Verification items for the finished model (mm, model axes). A direction names the side the tool comes from. Coordinates: 2 decimals unless noted, no trailing zeros. Loops run counter-clockwise (first coordinate to the right, second up) from the corner with the lowest first, then second, coordinate; pieces in that order, holes last. Notation, with made-up numbers: (-3, 73.25) -> (33, 73.25) arc R26 ccw to (33, 96.25) -> close; hole circle Ø10 at (7.25, 30). An arc over 180 degrees is marked (long way). Write item = value, one per line.
Autodesk Inventor part; units mm, degrees
ref_plane "YZ Plane" through (0, 0, 0) normal (1, 0, 0) x (0, 1, 0)
ref_plane "XZ Plane" through (0, 0, 0) normal (0, 1, 0) x (-1, 0, 0)
ref_plane "XY Plane" through (0, 0, 0) normal (0, 0, 1) x (1, 0, 0)
ref_plane "Work Plane2" through (0, 0, 0) normal (0, -1, 0) x (1, 0, 0)
sketch "Sketch33" plane through (0, 0, 0) normal (0, -1, 0) x (1, 0, 0)
  line L0 (74.8, -53.4338) -> (0, -53.4338)
  line L1 (0, -53.4338) -> (0, 0)
  line L2 (0, 0) -> (74.8, 0)
  line L3 (74.8, 0) -> (74.8, -53.4338)
  line L4 (74.8, -53.4338) -> (0, -53.4338)
  line L5 (0, -53.4338) -> (0, 0)
  line L6 (0, 0) -> (74.8, 0)
  line L7 (74.8, 0) -> (74.8, -53.4338)
  circle A0 centre (52, -49.5) radius 1.5
  circle A1 centre (52, -49.5) radius 1.5
  circle A2 centre (3, -47.2929) radius 1.5
  circle A3 centre (3, -47.2929) radius 1.5
  circle A4 centre (3, -15.7071) radius 1.5
  circle A5 centre (3, -15.7071) radius 1.5
  circle A6 centre (55, -2.5) radius 1.5
  circle A7 centre (55, -2.5) radius 1.5
  line L8 (74.8, -53.4338) -> (0, -53.4338)
  line L9 (0, -53.4338) -> (0, -58.4338)
  line L10 (0, -58.4338) -> (74.8, -58.4338)
  line L11 (74.8, -58.4338) -> (74.8, -53.4338)
  line L12 (0, -58.4338) -> (-5, -58.4338)
  line L13 (-5, -58.4338) -> (-5, -53.4338)
  line L14 (-5, -53.4338) -> (0, -53.4338)
  line L15 (0, -53.4338) -> (0, -58.4338)
  line L16 (0, 0) -> (-5, 0)
  line L17 (-5, 0) -> (-5, -53.4338)
  line L18 (-5, -53.4338) -> (0, -53.4338)
  line L19 (0, -53.4338) -> (0, 0)
  line L20 (-5, 0) -> (0, 0)
  line L21 (0, 0) -> (0, 5)
  line L22 (0, 5) -> (-5, 5)
  line L23 (-5, 5) -> (-5, 0)
  line L24 (0, 5) -> (74.8, 5)
  line L25 (74.8, 5) -> (74.8, 0)
  line L26 (74.8, 0) -> (0, 0)
  line L27 (0, 0) -> (0, 5)
  line L28 (74.8, -53.4338) -> (69.8, -53.4338)
  line L29 (69.8, -53.4338) -> (69.8, 5)
  line L30 (69.8, 5) -> (74.8, 5)
  line L31 (74.8, 5) -> (74.8, -53.4338)
  point P0 (74.8, 0)
  dimension "d220" = 5
  dimension "d221" = 5
  dimension "d222" = 5
  dimension "d223" = 5
extrude "Extrusion32" add sketch "Sketch33" along normal blind 5
ref_plane "Work Plane16" through (0, 0, 0) normal (0, 1, 0) x (1, 0, 0)
sketch "Sketch38" plane through (0, 0, 0) normal (0, 1, 0) x (1, 0, 0)
  line L0 (74.8, -5) -> (-5, -5)
  line L1 (-5, 58.4338) -> (74.8, 58.4338)
  line L2 (-5, -5) -> (-2, -5)
  line L3 (-2, -5) -> (-2, 58.4338)
  line L4 (-2, 58.4338) -> (-5, 58.4338)
  line L5 (-5, 58.4338) -> (-5, -5)
  line L6 (-5, -5) -> (-5, 58.4338)
  line L7 (74.8, 58.4338) -> (74.8, -5)
  line L8 (-5, 58.4338) -> (74.8, 58.4338)
  line L9 (74.8, 58.4338) -> (74.8, 55.4338)
  line L10 (74.8, 55.4338) -> (-5, 55.4338)
  line L11 (-5, 55.4338) -> (-5, 58.4338)
  line L12 (74.8, 58.4338) -> (71.8, 58.4338)
  line L13 (71.8, 58.4338) -> (71.8, 22.8825)
  line L14 (71.8, 22.8825) -> (74.8, 22.8825)
  line L15 (74.8, 22.8825) -> (74.8, 58.4338)
  line L16 (74.8, -5) -> (71.8, -5)
  line L17 (71.8, -5) -> (71.8, 10.5966)
  line L18 (71.8, 10.5966) -> (74.8, 10.5966)
  line L19 (74.8, 10.5966) -> (74.8, -5)
  line L20 (74.8, -5) -> (-5, -5)
  line L21 (-5, -5) -> (-5, -1.9965)
  line L22 (-5, -1.9965) -> (74.8, -1.9965)
  line L23 (74.8, -1.9965) -> (74.8, -5)
  point P0 (0, 0)
  point P1 (71.8, -1.9965)
  point P2 (-2, -1.9965)
  point P3 (-2, 55.4338)
  point P4 (71.8, 55.4338)
  dimension "d231" = 3
  dimension "d232" = 3
  dimension "d233" = 3
extrude "Extrusion33" add sketch "Sketch38" along normal blind 20 contours L0 L17 L22 L7 | L0 L3 L22 L17 | L22 L17 L18 L7 | L0 L5 L22 L3 | L22 L5 L10 L3 | L14 L13 L10 L7 | L10 L5 L1 L3 | L3 L1 L13 L10 | L10 L13 L1 L7
ref_plane "Work Plane11" through (71.8, 0, 1.9965) normal (0, 0, -1) x (-1, 0, 0)
sketch "Sketch45" plane through (71.8, 0, 1.9965) normal (0, 0, -1) x (-1, 0, 0)
  line L0 (47.3, 2) -> (47.3, 11)
  line L1 (73.8, 0) -> (0, 0)
  line L2 (47.3, 11) -> (45.8, 11)
  line L3 (45.8, 11) -> (45.8, 0)
  line L4 (45.8, 0) -> (47.3, 0)
  line L5 (47.3, 0) -> (47.3, 11)
  line L6 (47.3, 11) -> (45.8, 11)
  line L7 (45.8, 11) -> (45.8, 20.3018)
  line L8 (45.8, 20.3018) -> (47.3, 20.3018)
  line L9 (47.3, 20.3018) -> (47.3, 11)
  line L10 (68.3, 11) -> (47.3, 11)
  line L11 (47.3, 20.3018) -> (68.3, 20.3018)
  line L12 (68.3, 20.3018) -> (68.3, 11)
  line L13 (68.3, 11) -> (47.3, 11)
  line L14 (47.3, 11) -> (47.3, 20.3018)
  line L15 (45.8, 11) -> (19.8, 11)
  line L16 (19.8, 11) -> (19.8, 20.3018)
  line L17 (19.8, 20.3018) -> (45.8, 20.3018)
  line L18 (45.8, 20.3018) -> (45.8, 11)
  point P0 (71.8, 0)
  dimension "d243" = 1.5
  dimension "d244" = 26
extrude "Extrusion37" cut sketch "Sketch45" against normal blind 10 contours L9 L11 L12 L10 | L15 L16 L17 L7
ref_plane "Work Plane10" through (0, 20, 0) normal (0, 1, 0) x (1, 0, 0)
sketch "Sketch46" plane through (0, 20, 0) normal (0, 1, 0) x (1, 0, 0)
  line L0 (-2, 55.4338) -> (71.8, 55.4338)
  line L1 (75.7583, 22.3753) -> (69.7041, 22.3753)
  line L2 (69.7041, 22.3753) -> (69.7041, 55.4338)
  line L3 (69.7041, 55.4338) -> (75.7583, 55.4338)
  line L4 (75.7583, 55.4338) -> (75.7583, 22.3753)
  point P0 (0, 0)
extrude "Extrusion38" cut sketch "Sketch46" against normal blind 5
ref_plane "Work Plane14" through (0, 15, 0) normal (0, 1, 0) x (1, 0, 0)
sketch "Sketch47" plane through (0, 15, 0) normal (0, 1, 0) x (1, 0, 0)
  line L0 (70.1, 40.5) -> (70.1, 49.5)
  line L1 (70.1, 40.5) -> (76.1155, 40.5)
  line L2 (76.1155, 40.5) -> (76.1155, 49.5)
  line L3 (76.1155, 49.5) -> (70.1, 49.5)
  line L4 (70.1, 49.5) -> (70.1, 40.5)
  point P0 (0, 0)
  dimension "d249" = 9
extrude "Extrusion39" cut sketch "Sketch47" against normal blind 15
ref_plane "Work Plane9" through (0, 20, 0) normal (0, 1, 0) x (1, 0, 0)
sketch "Sketch48" plane through (0, 20, 0) normal (0, 1, 0) x (1, 0, 0)
  line L0 (74.8, 58.4338) -> (-5, 58.4338)
  line L1 (68.5228, 52.4259) -> (68.2069, 52.4259)
  line L2 (68.2069, 52.4259) -> (68.2069, 58.4338)
  line L3 (68.2069, 58.4338) -> (68.5228, 58.4338)
  line L4 (68.5228, 58.4338) -> (68.5228, 52.4259)
  line L5 (68.2069, 58.4338) -> (68.5228, 58.4338)
  line L6 (68.5228, 58.4338) -> (68.5228, 53.4262)
  line L7 (68.5228, 53.4262) -> (68.2069, 53.4262)
  line L8 (68.2069, 53.4262) -> (68.2069, 58.4338)
  line L9 (-2, 55.4338) -> (74.8, 55.4338)
  line L10 (68.5228, 55.4338) -> (50.5228, 55.4338)
  line L11 (50.5228, 55.4338) -> (50.5228, 58.4338)
  line L12 (50.5228, 58.4338) -> (68.5228, 58.4338)
  line L13 (68.5228, 58.4338) -> (68.5228, 55.4338)
  line L14 (51.9394, 55.4338) -> (3.9394, 55.4338)
  line L15 (3.9394, 55.4338) -> (3.9394, 58.4338)
  line L16 (3.9394, 58.4338) -> (51.9394, 58.4338)
  line L17 (51.9394, 58.4338) -> (51.9394, 55.4338)
  line L18 (-5, 58.4338) -> (-5, -5)
  line L19 (-5, 44.9754) -> (3.9394, 44.9754)
  line L20 (3.9394, 44.9754) -> (3.9394, 17.8349)
  line L21 (3.9394, 17.8349) -> (-5, 17.8349)
  line L22 (-5, 17.8349) -> (-5, 44.9754)
  line L23 (-5, 12.2802) -> (-0.5303, 12.2802)
  line L24 (-0.5303, 12.2802) -> (-0.5303, 2.9287)
  line L25 (-0.5303, 2.9287) -> (-5, 2.9287)
  line L26 (-5, 2.9287) -> (-5, 12.2802)
  point P0 (0, 0)
  point P1 (68.2069, 55.4338)
  dimension "d252" = 18
  dimension "d253" = 48
ref_plane "Work Plane8" through (0, 20, 0) normal (0, 1, 0) x (1, 0, 0)
sketch "Sketch49" plane through (0, 20, 0) normal (0, 1, 0) x (1, 0, 0)
  line L0 (74.8, 58.4338) -> (-5, 58.4338)
  line L1 (-2, 55.4338) -> (74.8, 55.4338)
  line L2 (50.5217, 58.4338) -> (3.9392, 58.4338)
  line L3 (3.9392, 58.4338) -> (3.9392, 55.4338)
  line L4 (3.9392, 55.4338) -> (50.5217, 55.4338)
  line L5 (50.5217, 55.4338) -> (50.5217, 58.4338)
  point P0 (0, 0)
extrude "Extrusion40" cut sketch "Sketch48" against normal blind 5 contours L23 L24 L25 L18 | L19 L20 L21 L18 | L2 L9 L17 L0 | L17 L9 L11 L0 | L11 L9 L15 L0
ref_plane "Work Plane13" through (26, 11, 1.9965) normal (0, 1, 0) x (1, 0, 0)
sketch "Sketch50" plane through (26, 11, 1.9965) normal (0, 1, 0) x (1, 0, 0)
  line L0 (-1.5, 0) -> (-1.5, -3.0035)
  line L1 (-31, -3.0035) -> (-22.5, -3.0035)
  line L2 (-1.5, 0) -> (-22.5, 0)
  line L3 (-22.5, 0) -> (-22.5, -3.0035)
  line L4 (-22.5, -3.0035) -> (-1.5, -3.0035)
  line L5 (-1.5, -3.0035) -> (-1.5, 0)
  line L6 (0, 0) -> (0, -3.0035)
  line L7 (26, 0) -> (26, -3.0035)
  line L8 (0, -3.0035) -> (26, -3.0035)
  line L9 (26, -3.0035) -> (26, 0)
  line L10 (26, 0) -> (0, 0)
  line L11 (0, 0) -> (0, -3.0035)
  point P0 (-26, 1.9965)
  point P1 (26, -3.0035)
extrude "Extrusion41" add sketch "Sketch50" along normal blind 5
sketch "Sketch51" plane through (0, 20, 0) normal (0, 1, 0) x (1, 0, 0)
  point P0 (0, 0)
sketch "Sketch52" plane through (0, 20, 0) normal (0, 1, 0) x (1, 0, 0)
  line L0 (3.9394, 58.4338) -> (-5, 58.4338)
  line L1 (-5, -5) -> (3.5, -5)
  line L2 (74.8, 55.4338) -> (74.8, 49.5)
  line L3 (-5, 58.4338) -> (-5, 44.9754)
  line L4 (74.8, 55.4338) -> (74.8, 58.4338)
  line L5 (68.2069, 58.4338) -> (68.2069, 55.4338)
  line L6 (74.8, -5) -> (74.8, 10.5966)
  line L7 (52, -1.9965) -> (52, -5)
  line L8 (52, -5) -> (74.8, -5)
  line L9 (71.8, -1.9965) -> (52, -1.9965)
  line L10 (71.8, 10.5966) -> (71.8, -1.9965)
  line L11 (26, -5) -> (26, -1.9965)
  line L12 (24.5, -1.9965) -> (24.5, -5)
  line L13 (3.5, -5) -> (3.5, -1.9965)
  line L14 (-5, 12.2802) -> (-2, 12.2802)
  line L15 (-2, 2.9287) -> (-5, 2.9287)
  point P0 (0, 0)
  dimension "d258" = 63.4338
  dimension "d259" = 79.8
  dimension "d260" = 6.5931
  dimension "d261" = 3
  dimension "d262" = 22.8
  dimension "d263" = 3.0035
  dimension "d264" = 3
  dimension "d265" = 12.593
  dimension "d266" = 15.5966
  dimension "d267" = 19.8
  dimension "d268" = 26
  dimension "d269" = 21
  dimension "d270" = 8.5
  dimension "d271" = 9.3515
  dimension "d272" = 13.4584
  dimension "d273" = 8.9394
properties part number "_3DPrint"
1) Release check for a two-part mould opening along Z. For faces 4 (the face through (-3, 18, -2.929)), 5 (the face through (36, 15, -57)) record: pulls with the +Z half, pulls with the -Z half, needs draft (parallel to the pull), parting line crosses it, or undercut.
Ans:
face_4 = undercut
face_5 = needs draft
2) Material ranges on line 1 (Z direction, x = 3, y = -2.05); line 2 (X direction, y = 11.25, z = -34); line 3 (Z direction, x = 52.5, y = 12), recorded low to high.
Ans:
line_1 = -58.43 to -48.79, -45.79 to -17.21, -14.21 to 5
line_2 = -5 to -2, 71.8 to 74.8
line_3 = -58.43 to -55.43, 2 to 5
3) Depth check by flat-ended pin: pin 1 Ø1.5 at (x, z) = (33, 4) entering from +Y; pin 2 Ø0.9 at (x, z) = (73, -31.5) entering from +Y; pin 3 Ø10 at (x, z) = (33, -12.5) entering from +Y. Enter the tip coordinate at first touch or a pass-through.
Ans:
pin_1 = 16
pin_2 = 15
pin_3 = 0
4) Sectioned sample at D-D, the plane x = 16.5. Record the cut outline in (y, z), plus the area to 3 significant figures.
Ans:
outline = (-5, -58.43) -> (15, -58.43) -> (15, -55.43) -> (0, -55.43) -> (0, 2) -> (16, 2) -> (16, 5) -> (-5, 5) -> close
area = 410 mm2
5) Sectioned sample at B-B, the plane y = 6.5. Record the cut outline in (x, z).
Ans:
outline = (-5, -58.43) -> (74.8, -58.43) -> (74.8, -49.5) -> (71.8, -49.5) -> (71.8, -55.43) -> (-2, -55.43) -> (-2, 2) -> (71.8, 2) -> (71.8, -10.6) -> (74.8, -10.6) -> (74.8, 5) -> (-5, 5) -> close; (71.8, -40.5) -> (74.8, -40.5) -> (74.8, -22.88) -> (71.8, -22.88) -> close
6) Sectioned sample at A-A, the plane x = 55. Record the cut outline in (y, z).
Ans:
outline = (-5, -58.43) -> (15, -58.43) -> (15, -55.43) -> (0, -55.43) -> (0, -4) -> (-5, -4) -> close; (-5, -1) -> (0, -1) -> (0, 2) -> (20, 2) -> (20, 5) -> (-5, 5) -> close
7) Tool access check on faces 1 (the face through (73, 8, -49.5)), 2 (the face through (-4, 15, -8)), 3 (the face through (36, 8, -55.434)). Record the directions out of +Z, -Z, +X, -X, +Y, -Y that give a thin tool (end or side, any length) a straight path to the whole face; none if there is none.
Ans:
face_1 = +X, +Y
face_2 = -X, +Y
face_3 = +Y
8) Sectioned sample at C-C, the plane z = -6. Record the cut outline in (x, y).
Ans:
outline = (-5, -5) -> (74.8, -5) -> (74.8, 20) -> (71.8, 20) -> (71.8, 0) -> (-2, 0) -> (-2, 15) -> (-5, 15) -> close
